For this review, take the finished solid that the model builds, in its own axes (mm). Face numbers are marked on the shaded views. A direction names the side the tool comes from. Round coordinates to 2 decimals unless told otherwise and drop trailing zeros. Loops run counter-clockwise (first coordinate to the right, second up) from the corner with the lowest first, then second, coordinate; pieces in that order, holes last.
1) Take a section at A-A (y = 17). State the section outline as (x, z) points.
2) Tool access review of the marked faces 4, 5 and 6: name each direction out of +Z, -Z, +X, -X, +Y, -Y from which nothing blocks a thin tool from reaching the whole face with its end or side.
3) Insertion check: pin 1 (2 mm diameter, centred on y = 28, z = -12, fed in from -X); pin 2 (4 mm diameter, centred on y = 16.5, z = -37.5, fed in from +X). Each pin has a flat end and moves straight along its axis. Give the tip position at first contact, or say it passes through.
4) Take a section at C-C (z = -13.5). State the section outline as (x, y) points.
5) Wall thickness on L1, parallel to X at y = 8.5, z = -40; L2, parallel to Z at x = -92, y = 18: over which ranges is each line inside the solid? List them lowest first.
6) Take a section at B-B (x = -26). State the section outline as (y, z) points.
7) Mouldability with a two-part tool opening along X and no side actions: class the marked faces 1, 2 and 3 as pulls with the +X half, pulls with the -X half, needs draft (parallel to the pull), parting line crosses it, or undercut.
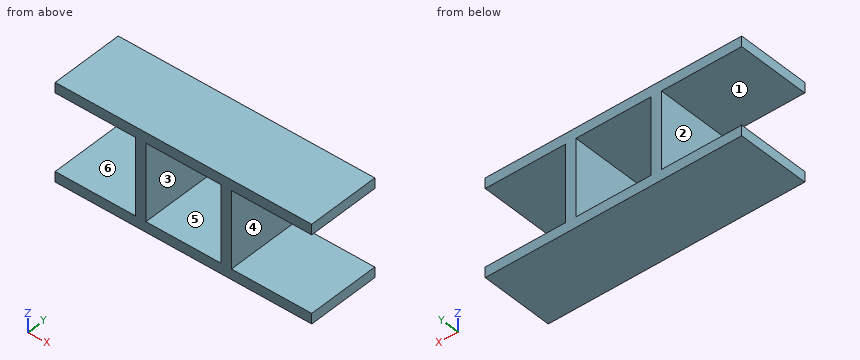
Autodesk Inventor part; units mm, degrees
ref_plane "YZ Plane" through (0, 0, 0) normal (1, 0, 0) x (0, 1, 0)
ref_plane "XZ Plane" through (0, 0, 0) normal (0, 1, 0) x (-1, 0, 0)
ref_plane "XY Plane" through (0, 0, 0) normal (0, 0, 1) x (1, 0, 0)
sketch "Sketch1" plane through (0, 0, 0) normal (0, 1, 0) x (-1, 0, 0)
  line L0 (0, 0) -> (123.5, 0)
  line L1 (123.5, 0) -> (123.5, -5)
  line L2 (123.5, -5) -> (0, -5)
  line L3 (0, -5) -> (0, 0)
  line L4 (0, -47.1) -> (123.5, -47.1)
  line L5 (123.5, -47.1) -> (123.5, -42.1)
  line L6 (123.5, -42.1) -> (0, -42.1)
  line L7 (0, -42.1) -> (0, -47.1)
  dimension "d0" = 123.5
  dimension "d1" = 5
  dimension "d2" = 123.5
  dimension "d3" = 5
  dimension "d4" = 47.1
  dimension "d7" = 0
extrude "Extrusion1" add sketch "Sketch1" along normal blind 35
sketch "Sketch2" plane through (0, 35, 0) normal (0, 1, 0) x (1, 0, 0)
  line L0 (-123.5, 0) -> (0, 0)
  line L1 (0, 0) -> (0, 5)
  line L2 (0, 5) -> (-123.5, 5)
  line L3 (-123.5, 5) -> (-123.5, 0)
  line L4 (0, 47.1) -> (-123.5, 47.1)
  line L5 (-123.5, 47.1) -> (-123.5, 42.1)
  line L6 (-123.5, 42.1) -> (0, 42.1)
  line L7 (0, 42.1) -> (0, 47.1)
  line L8 (-38.6667, 5) -> (-43.6667, 5)
  line L9 (-43.6667, 5) -> (-43.6667, 42.1)
  line L10 (-43.6667, 42.1) -> (-38.6667, 42.1)
  line L11 (-38.6667, 42.1) -> (-38.6667, 5)
  line L12 (-123.5, 42.1) -> (0, 42.1)
  line L13 (-84.8333, 5) -> (-79.8333, 5)
  line L14 (-79.8333, 5) -> (-79.8333, 42.1)
  line L15 (-79.8333, 42.1) -> (-84.8333, 42.1)
  line L16 (-84.8333, 42.1) -> (-84.8333, 5)
  dimension "d8" = 5
  dimension "d9" = 5
  dimension "d10" = 38.6667
  dimension "d11" = 38.6667
extrude "Extrusion2" add sketch "Sketch2" against normal blind 35 contours L16 L6 L14 L2 | L2 L9 L6 L11
properties part number "Parametric"
Response:
1. outline: (-123.5, -47.1) - (0, -47.1) - (0, -42.1) - (-38.67, -42.1) - (-38.67, -5) - (0, -5) - (0, 0) - (-123.5, 0) - (-123.5, -5) - (-84.83, -5) - (-84.83, -42.1) - (-123.5, -42.1) - close; hole (-79.83, -42.1) - (-43.67, -42.1) - (-43.67, -5) - (-79.83, -5) - close
2. face 4: +X, +Y, -Y
2. face 5: +Y, -Y
2. face 6: -X, +Y, -Y
3. pin 1: stops at x = -84.83
3. pin 2: stops at x = -38.67
4. outline: (-84.83, 0) - (-79.83, 0) - (-79.83, 35) - (-84.83, 35) - close; (-43.67, 0) - (-38.67, 0) - (-38.67, 35) - (-43.67, 35) - close
5. L1: x = -84.83 to -79.83, -43.67 to -38.67
5. L2: z = -47.1 to -42.1, -5 to 0
6. outline: (0, -47.1) - (35, -47.1) - (35, -42.1) - (0, -42.1) - close; (0, -5) - (35, -5) - (35, 0) - (0, 0) - close
7. face 1: needs draft
7. face 2: pulls with the -X half
7. face 3: undercut
